The figure shows three views and two pictorial views of one solid part (mm, origin at its lowest corner). Answer the questions. Coordinates: 2 decimals unless noted, no trailing zeros. Loops run counter-clockwise (first coordinate to the right, second up) from the corner with the lowest first, then second, coordinate; pieces in that order, holes last.
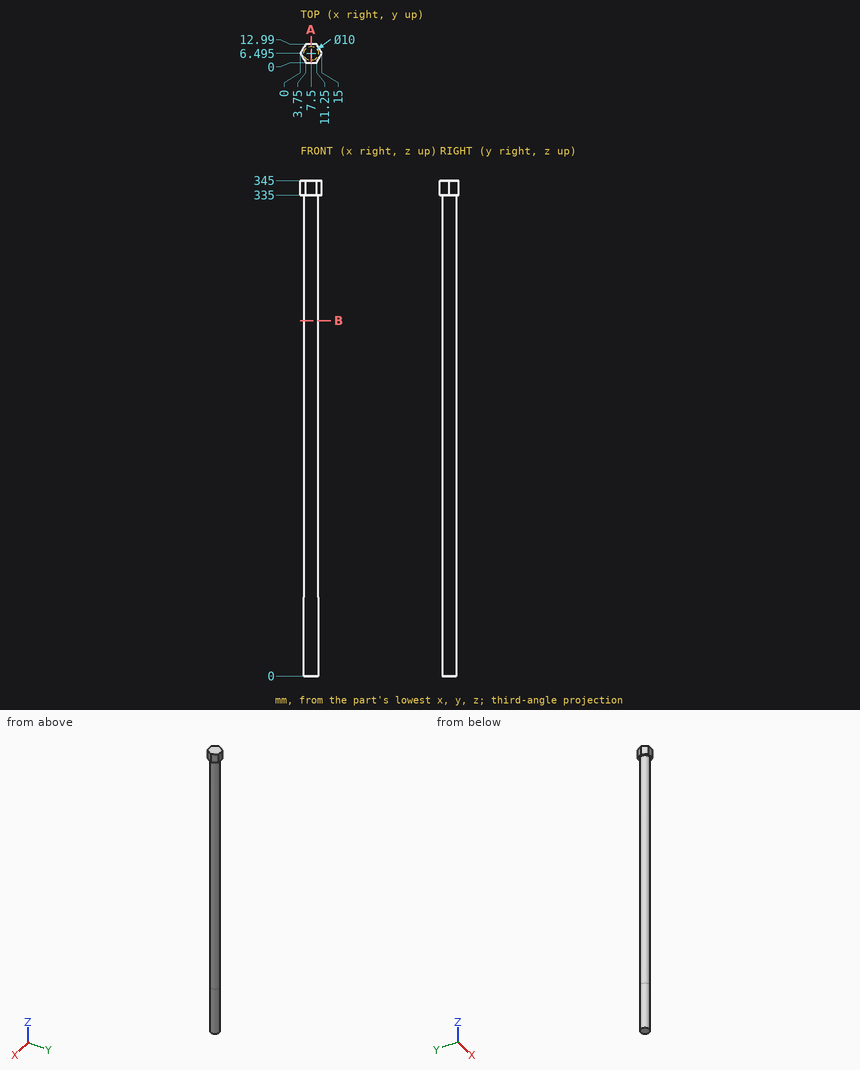
Q1. Straight lines are drawn through the part: probe 1 along Z at (x, y) = (9.5, 1.5); probe 2 along X at (y, z) = (3.25, 64) (1 decimal); probe 3 along X at (y, z) = (6.5, 325.5). For each, find the intervals that lie inside material, in ascending order.
Findings below:
probe 1: z = 335 to 345
probe 2: x = 3.7 to 11.3
probe 3: x = 2.5 to 12.5
Q2. A cutting plane is placed at B-B (z = 247.5). Give the vertices of the cut face in (x, y) (1 decimal).
Findings below:
outline: circle Ø10 at (7.5, 6.5)
Q3. Flat-ended cylindrical pins translate along their axes: pin 1 Ø4 at (y, z) = (4, 257) entering from +X (1 decimal); pin 2 Ø4 at (x, y) = (9, 7) entering from -Z; pin 3 Ø6 at (x, z) = (9.5, 249) entering from -Y (1 decimal); pin 4 Ø2 at (x, z) = (2, 301) entering from -Y (1 decimal). Find the tip coordinate at first contact, or state that the pin passes through.
Findings below:
pin 1: stops at x = 12.5
pin 2: stops at z = 0
pin 3: stops at y = 1.5
pin 4: stops at y = 4.3
Q4. A cutting plane is placed at A-A (x = 7.5). Give the vertices of the cut face in (y, z) (1 decimal).
Findings below:
outline: (0, 335) - (1.5, 335) - (1.5, 0) - (11.5, 0) - (11.5, 335) - (13, 335) - (13, 345) - (0, 345) - close
